Source: CAD feature listing. Evaluate the final solid. Frame: model axes, mm. A direction names the side the tool comes from. Give positions to 0.01 mm unless a question says otherwise; leave off trailing zeros. Loops run counter-clockwise (first coordinate to the right, second up) from the corner with the lowest first, then second, coordinate; pieces in that order, holes last. Notation, with made-up numbers: (50, 17) - (77, 17) arc R14 ccw to (77, 28) - close; hole circle Ø10 at (-38, 55.25). An arc over 180 degrees is marked (long way). Write each question's results on one line, items separated by ' | '. Start each with the question number.
(1) Cut plane D-D on y = 7. Return the cut outline in (x, z), then the cut area to 3 significant figures.
(2) Cut plane C-C on x = -4. Return the cut outline in (y, z), then the cut area to 3 significant figures.
(3) Cut plane A-A on z = 0. Return the cut outline in (x, y), then the cut area to 3 significant figures.
(4) Pull-direction query (X, two-part tool) for faces 1 (the cylindrical face through (40.17, 4.93, 32.5)), 2 (the cylindrical face through (-34.89, 4.93, 35.38)), 3 (the cylindrical face through (4.05, 4.93, 18.78)); classes: pulls with the +X half, pulls with the -X half, needs draft (parallel to the pull), parting line crosses it, or undercut.
(5) Material intervals for line 1 along Z through (x, y) = (0, 7); line 2 along X through (y, z) = (8.75, 24.5); line 3 along Z through (x, y) = (-38, 3.25), sorted ascending. Write a range as [from, to].
(6) Reachability of faces 4 (the cylindrical face through (26, 5, 0)), 5 (the cylindrical face through (-35.16, 4.93, -35.26)), 6 (the flat face through (-18, 5, 12.5)) from +Z, -Z, +X, -X, +Y, -Y: full face, straight path, thin tool, end or side. Return the list, or none.
(7) Contact query for flat-ended pins moving along their axis: pin 1 (3 mm diameter, centred on x = -26.5, y = 6.5, fed in from +Z); pin 2 (2 mm diameter, centred on y = 7.5, z = -9.5, fed in from -X); pin 3 (3 mm diameter, centred on y = 5.5, z = 17.5, fed in from +X). Output: stop coordinate, or through.
(8) Cut plane B-B on x = 35. Return the cut outline in (y, z).
Autodesk Inventor part; units mm, degrees
ref_plane "YZ Plane" through (0, 0, 0) normal (1, 0, 0) x (0, 1, 0)
ref_plane "XZ Plane" through (0, 0, 0) normal (0, 1, 0) x (-1, 0, 0)
ref_plane "XY Plane" through (0, 0, 0) normal (0, 0, 1) x (1, 0, 0)
sketch "Sketch1" plane through (0, 0, 0) normal (0, 1, 0) x (-1, 0, 0)
  arc A0 (-50.2663, 19.7308) -> (-50.2663, -19.7308) centre (0, 0) ccw
  line L0 (24.8197, 37.5) -> (-24.2023, 37.5)
  line L1 (-24.2023, -37.5) -> (24.8197, -37.5)
  circle A1 centre (0, 0) radius 12.5
  circle A2 centre (0, -22.5) radius 5.5
  circle A3 centre (0, 22.5) radius 5.5
  arc A4 (-24.2023, 37.5) -> (-50.2663, 19.7308) centre (-24.2023, 9.5) ccw
  line L2 (-14, 0) -> (-38, 0)
  arc A5 (-50.2663, -19.7308) -> (-24.2023, -37.5) centre (-24.2023, -9.5) ccw
  line L3 (0, 0) -> (-36.2595, -20.9344)
  line L4 (0, 0) -> (-38.6065, 22.2895)
  circle A6 centre (-27.7128, 16) radius 6
  circle A7 centre (-27.7128, -16) radius 6
  arc A8 (-22.5167, 13) -> (-22.5167, -13) centre (0, 0) ccw
  arc A9 (-32.909, 19) -> (-32.909, -19) centre (0, 0) ccw
  line L5 (38.0847, -33.6906) -> (38.0847, -32.2803)
  line L6 (38.0847, 32.2803) -> (38.0847, 33.6906)
  arc A10 (36, 12.5) -> (43.4536, 29.1667) centre (36, 22.5) ccw
  arc A11 (43.4536, -29.1667) -> (36, -12.5) centre (36, -22.5) ccw
  line L7 (0, 12.5) -> (0, -12.5)
  arc A12 (3.9746, 26.3016) -> (3.6179, 25.7471) centre (24.8197, 12.5) ccw
  arc A13 (-0.1803, 12.4987) -> (0, 9.5026) centre (24.8197, 12.5) ccw
  arc A14 (1.3171, -21.0223) -> (3.9746, -26.3016) centre (24.8197, -12.5) ccw
  arc A15 (24.8197, -37.5) -> (43.4536, -29.1667) centre (24.8197, -12.5) ccw
  arc A16 (0, -9.5026) -> (-0.1803, -12.4987) centre (24.8197, -12.5) ccw
  arc A17 (43.4536, 29.1667) -> (24.8197, 37.5) centre (24.8197, 12.5) ccw
  line L8 (0, 12.5) -> (36, 12.5)
  line L9 (49.8197, 12.5) -> (55, 12.5)
  line L10 (0, -12.5) -> (36, -12.5)
  line L11 (49.8197, -12.5) -> (57, -12.5)
  arc A18 (24.8197, -12.5) -> (29.6533, -12.0283) centre (24.8197, 12.5) ccw
  arc A19 (36.8095, -9.4373) -> (38.0847, -8.6906) centre (24.8197, 12.5) ccw
  arc A20 (-24.2389, 20.892) -> (-27.7128, 16) centre (0, 0) ccw
  arc A21 (-30.2125, -10.5455) -> (-24.2389, -20.892) centre (0, 0) ccw
  circle A22 centre (36, 22.5) radius 5.5
  circle A23 centre (36, -22.5) radius 5.5
  dimension "d5" = 11
  dimension "d6" = 11
  dimension "d0" = 108
  dimension "d4" = 25
  dimension "d7" = 45
  dimension "d8" = 22.5
  dimension "d9" = 37.5
  dimension "d10" = 37.5
  dimension "d13" = 30
  dimension "d14" = 30
  dimension "d15" = 12
  dimension "d16" = 12
  dimension "d17" = 20
  dimension "d18" = 20
  dimension "d19" = 36
  dimension "d20" = 36
  dimension "d23" = 11
  dimension "d24" = 11
extrude "Extrusion1" add sketch "Sketch1" along normal blind 10 contours A4 L0 A17 A10 L8 A1 L4 A6 A9 A7 L3 L10 A11 A15 L1 A5 A0 | A1 L3 A8 L4
equation "\"d5\" = d6"
equation "\"d16\" = d15"
equation "\"d18\" = d17"
Ans:
1) outline: (-43.45, -29.17) arc R25 ccw to (-24.82, -37.5) - (24.2, -37.5) arc R28 ccw to (50.27, -19.73) arc R54 ccw to (50.27, 19.73) arc R28 ccw to (24.2, 37.5) - (-24.82, 37.5) arc R25 ccw to (-43.45, 29.17) arc R10 ccw to (-36, 12.5) - (0, 12.5) arc R12.5 cw to (0, -12.5) - (-36, -12.5) arc R10 ccw to start; hole circle Ø11 at (-36, -22.5); hole circle Ø11 at (-36, 22.5); hole circle Ø11 at (0, -22.5); hole circle Ø11 at (0, 22.5); hole (22.52, -13) arc R6 ccw to (32.91, -19) arc R38 ccw to (32.91, 19) arc R6 ccw to (22.52, 13) arc R26 cw to start | area: 4,580 mm^2
2) outline: (0, -37.5) - (10, -37.5) - (10, -26.27) - (0, -26.27) - close; (0, -18.73) - (10, -18.73) - (10, -12.5) - (0, -12.5) - close; (0, 12.5) - (10, 12.5) - (10, 18.73) - (0, 18.73) - close; (0, 26.27) - (10, 26.27) - (10, 37.5) - (0, 37.5) - close | area: 349 mm^2
3) outline: (12.5, 0) - (26, 0) - (26, 10) - (12.5, 10) - close; (38, 0) - (54, 0) - (54, 10) - (38, 10) - close | area: 295 mm^2
4) face 1: pulls with the +X half | face 2: pulls with the -X half | face 3: undercut
5) line 1: [-37.5, -28], [-17, -12.5], [12.5, 17], [28, 37.5] | line 2: [-45.8, -41.12], [-30.88, -5.12], [5.12, 47.85] | line 3: [-33.74, -27.62], [-17.38, -12.7], [12.7, 17.38], [27.62, 33.74]
6) face 4: +Y, -Y | face 5: -Z, -X, +Y, -Y | face 6: -X, +Y, -Y
7) pin 1: z = 37.5 | pin 2: x = 6.78 | pin 3: x = 51.58
8) outline: (0, -35.33) - (10, -35.33) - (10, -14.8) - (0, -14.8) - close; (0, 14.8) - (10, 14.8) - (10, 35.33) - (0, 35.33) - close
